Design review of the part built by this model. Coordinates are the model's own, in mm. A direction names the side the tool comes from. Round coordinates to 2 decimals unless told otherwise and drop trailing zeros. Loops run counter-clockwise (first coordinate to the right, second up) from the corner with the lowest first, then second, coordinate; pieces in that order, holes last. Notation, with made-up numbers: M 25.5,12.25 L 62.5,12.25 A5 ccw 62.5,20.25 Z; hole C -36.5,-8 d6. An arc over 180 degrees is marked long. One line per item, written item: value. Start each with the question number.
Item 1: Mouldability with a two-part tool opening along Y and no side actions: class faces 4 (the flat face through (0, 76, 6)), 5 (the cylindrical face through (1, 40, 0)), 6 (the flat face through (1, 70, 18.5)), 7 (the flat face through (1, 101, 12.5)) as released by +Y, released by -Y, zero draft, split by the parting line, or undercut.
Item 2: For line 1 along Y through (x, z) = (1.5, 12); line 2 along Z through (x, y) = (1, 64.5); line 3 along Z through (x, y) = (0.8, 115), list the stretches that pass through material, from the lowest coordinate up.
Item 3: Clearance check with flat-ended pins moving along their axes: pin 1 (6 mm diameter, centred on y = 80, z = 11, fed in from +X); pin 2 (1.8 mm diameter, centred on y = 115, z = 12, fed in from -X); pin 3 (1.5 mm diameter, centred on x = 5.5, z = 7.5, fed in from -Y); pin 4 (1 mm diameter, centred on x = 7.5, z = 10, fed in from +Y). State where each tip first meets the part, or that it passes through.
Item 4: We need section B-B (x = 5). Write out the cut boundary in (y, z), then the cut area to 3 significant figures.
Item 5: We need section A-A (z = 0). Write out the cut boundary in (x, y), then the cut area to 3 significant figures.
Item 6: We need section C-C (z = 15.5). Write out the cut boundary in (x, y), then the cut area to 3 significant figures.
Item 7: We need section D-D (y = 104). Write out the cut boundary in (x, z), then the cut area to 3 significant figures.
Item 8: For faces 1 (the cylindrical face through (7.07, 46.69, 6.54)), 2 (the cylindrical face through (0.99, 30.07, -29.13)), 3 (the cylindrical face through (1, 94.2, -15.6)), list the 3-axis set-ups (+Z, -Z, +X, -X, +Y, -Y) from which the entire face can be reached by the end or side of a thin tool; tool diameter is ignored.
from build123d import *

# Parameters (mm, degrees)
SKETCH1_R           = 1.5
BOSS_EXTRUDE1_DEPTH = 2
SKETCH2_R           = 1.5
BOSS_EXTRUDE2_DEPTH = 10
FILLET1_R           = 2


with BuildPart() as part:
    # Sketch1 → Boss-Extrude1 (new body)
    with BuildSketch(Plane(origin=(0, 0, 0), x_dir=(0, 0, -1), z_dir=(1, 0, 0))):
        with BuildLine():
            Line((-25.968110327, 120), (25.968110327, 120))
            ThreePointArc((25.968110327, 120), (29.67212348, 76.455251784), (30.833602138, 32.768688884))
            ThreePointArc((30.833602138, 32.768688884), (29.089961469, 30.052105348), (25.891732052, 30.48964105))
            ThreePointArc((25.891732052, 30.48964105), (0, 40), (-25.891732052, 30.48964105))
            ThreePointArc((-25.891732052, 30.48964105), (-29.089961469, 30.052105348), (-30.833602138, 32.768688884))
            ThreePointArc((-30.833602138, 32.768688884), (-29.67212348, 76.455251784), (-25.968110327, 120))
        make_face()
        with Locations((-12, 115)):
            Circle(SKETCH1_R, mode=Mode.SUBTRACT)
        with Locations((12, 115)):
            Circle(SKETCH1_R, mode=Mode.SUBTRACT)
        with Locations((-12, 48)):
            Circle(SKETCH1_R, mode=Mode.SUBTRACT)
        with Locations((12, 48)):
            Circle(SKETCH1_R, mode=Mode.SUBTRACT)
        with BuildLine():
            Line((8, 89.7), (8, 81.7))
            ThreePointArc((8, 81.7), (0, 73.7), (-8, 81.7))
            Line((-8, 81.7), (-8, 89.7))
            ThreePointArc((-8, 89.7), (0, 97.7), (8, 89.7))
        make_face(mode=Mode.SUBTRACT)
        with BuildLine():
            Line((18.5, 105.2), (18.5, 97.2))
            ThreePointArc((18.5, 97.2), (15.5, 94.2), (12.5, 97.2))
            Line((12.5, 97.2), (12.5, 105.2))
            ThreePointArc((12.5, 105.2), (15.5, 108.2), (18.5, 105.2))
        make_face(mode=Mode.SUBTRACT)
        with BuildLine():
            Line((18.5, 74.2), (18.5, 66.2))
            ThreePointArc((18.5, 66.2), (15.5, 63.2), (12.5, 66.2))
            Line((12.5, 66.2), (12.5, 74.2))
            ThreePointArc((12.5, 74.2), (15.5, 77.2), (18.5, 74.2))
        make_face(mode=Mode.SUBTRACT)
        with BuildLine():
            Line((-12.5, 105.2), (-12.5, 97.2))
            ThreePointArc((-12.5, 97.2), (-15.5, 94.2), (-18.5, 97.2))
            Line((-18.5, 97.2), (-18.5, 105.2))
            ThreePointArc((-18.5, 105.2), (-15.5, 108.2), (-12.5, 105.2))
        make_face(mode=Mode.SUBTRACT)
        with BuildLine():
            Line((-12.5, 74.2), (-12.5, 66.2))
            ThreePointArc((-12.5, 66.2), (-15.5, 63.2), (-18.5, 66.2))
            Line((-18.5, 66.2), (-18.5, 74.2))
            ThreePointArc((-18.5, 74.2), (-15.5, 77.2), (-12.5, 74.2))
        make_face(mode=Mode.SUBTRACT)
    extrude(amount=BOSS_EXTRUDE1_DEPTH)

    # Sketch2 → Boss-Extrude2 (add)
    with BuildSketch(Plane(origin=(2, 0, 0), x_dir=(0, 0, -1), z_dir=(1, 0, 0))):
        with BuildLine():
            Line((-6.910390688, 49), (7.101020514, 49))
            ThreePointArc((7.101020514, 49), (17, 48), (7.101020514, 47))
            Line((7.101020514, 47), (-6.910390688, 47))
            ThreePointArc((-6.910390688, 47), (-17.186918444, 48), (-6.910390688, 49))
        make_face()
        with Locations((-12, 48)):
            Circle(SKETCH2_R, mode=Mode.SUBTRACT)
        with Locations((12, 48)):
            Circle(SKETCH2_R, mode=Mode.SUBTRACT)
    extrude(amount=BOSS_EXTRUDE2_DEPTH)

    # Fillet1
    fillet1_edges = [part.edges().sort_by_distance(p)[0] for p in [
        (7, 49, 6.910390688),
        (7, 47, 6.910390688),
        (7, 47, -7.101020514),
        (7, 49, -7.101020514),
    ]]
    fillet(fillet1_edges, radius=FILLET1_R)


solid = part.part
A:
1. face 4: zero draft
1. face 5: released by -Y
1. face 6: undercut
1. face 7: undercut
2. line 1: 38.16 to 46.5, 49.5 to 113.5, 116.5 to 120
2. line 2: -30.24 to -17.97, -13.03 to 13.03, 17.97 to 30.24
2. line 3: -26.52 to -13.5, -10.5 to 10.5, 13.5 to 26.52
3. pin 1: x = 2
3. pin 2: through
3. pin 3: y = 44.42
3. pin 4: y = 52.97
4. outline: M 45.83,7.29 A2 cw 47,5.47 L 47,-5.68 A2 cw 45.86,-7.48 A5 ccw long 50.14,-7.48 A2 cw 49,-5.68 L 49,5.47 A2 cw 50.17,7.29 A5.19 ccw long Z; hole C 48,-12 d3; hole C 48,12 d3
4. area: 178 mm2
5. outline: M 0,40 L 2,40 L 2,47 L 12,47 L 12,49 L 2,49 L 2,73.7 L 0,73.7 Z; M 0,97.7 L 2,97.7 L 2,120 L 0,120 Z
5. area: 132 mm2
6. outline: M 0,36.87 L 2,36.87 L 2,44.17 L 12,44.17 L 12,51.83 L 2,51.83 L 2,63.2 L 0,63.2 Z; M 0,77.2 L 2,77.2 L 2,94.2 L 0,94.2 Z; M 0,108.2 L 2,108.2 L 2,120 L 0,120 Z
6. area: 187 mm2
7. outline: M 0,-27.63 L 2,-27.63 L 2,-18.5 L 0,-18.5 Z; M 0,-12.5 L 2,-12.5 L 2,12.5 L 0,12.5 Z; M 0,18.5 L 2,18.5 L 2,27.63 L 0,27.63 Z
7. area: 86.5 mm2
8. face 1: +X, -Y
8. face 2: +X, -X, -Y
8. face 3: +X, -X
